Check sheet for the modelled part. Datum: model origin and axes. Units: mm. A direction names the side the tool comes from. Coordinates: 2 decimals unless noted, no trailing zeros. Order: outer loops, then holes, each group sorted by start corner. A loop starts at its lowest first (then second) coordinate and runs counter-clockwise, first axis right, second up.
from build123d import *

# Parameters (mm, degrees)
F0_W     = 115
F0_H     = 67
F1_DEPTH = 52
F2_T     = -2
F3_R     = 3
F5_DEPTH = 115
F6_W     = 25
F6_H     = 15
F7_DEPTH = 2
F9_DEPTH = 2


with BuildPart() as f1:
    # F0 (on Top) → F1 (new body)
    with BuildSketch(Plane.XY):
        Rectangle(F0_W, F0_H)
    extrude(amount=F1_DEPTH)

    # F2
    f2_openings = [f1.faces().sort_by_distance(p)[0] for p in [
        (0, 0, 52),
    ]]
    offset(amount=F2_T, openings=f2_openings)

    # F3
    f3_edges = [f1.edges().sort_by_distance(p)[0] for p in [
        (57.5, 33.5, 26),
        (57.5, -33.5, 26),
        (-57.5, -33.5, 26),
        (-57.5, 33.5, 26),
        (-57.5, 0, 0),
        (0, -33.5, 0),
        (0, 33.5, 0),
        (57.5, 0, 0),
    ]]
    fillet(f3_edges, radius=F3_R)

    # F4 (on face) → F5 (cut, through all)
    with BuildSketch(Plane(origin=(-57.5, 0, 0), x_dir=(0, -1, 0), z_dir=(-1, 0, 0))):
        with BuildLine():
            Line((-8.5, 52), (-18.5, 52))
            Line((-18.5, 52), (-18.5, 37))
            ThreePointArc((-18.5, 37), (-8.5, 27), (1.5, 37))
            Line((1.5, 37), (1.5, 52))
            Line((1.5, 52), (-8.5, 52))
        make_face()
    extrude(amount=-F5_DEPTH, mode=Mode.SUBTRACT)

    # F6 (on face) → F7 (cut, through all)
    with BuildSketch(Plane.YZ.offset(57.5)):
        with Locations((-14, 44.5)):
            Rectangle(F6_W, F6_H)
    extrude(amount=-F7_DEPTH, mode=Mode.SUBTRACT)

    # F8 (on face) → F9 (cut, through all)
    with BuildSketch(Plane.XZ.offset(33.5)):
        with BuildLine():
            Line((46, 52), (33, 52))
            Line((33, 52), (33, 43))
            ThreePointArc((33, 43), (33.5857864376, 41.5857864376), (35, 41))
            Line((35, 41), (44, 41))
            ThreePointArc((44, 41), (45.4142135624, 41.5857864376), (46, 43))
            Line((46, 43), (46, 52))
        make_face()
    extrude(amount=-F9_DEPTH, mode=Mode.SUBTRACT)


solid = f1.part
(1) Release check for a two-part mould opening along Y. For faces 3 (the flat face through (-55.5, 0, 27)), 4 (the cylindrical face through (56.6, -32.64, 27.84)), 5 (the flat face through (53, -32, 52)) record: +Y half, -Y half, draft (parallel to the pull), parting line (faces both ways), or undercut.
Filled in:
face 3: undercut
face 4: -Y half
face 5: draft
(2) Tool access check on faces 1 (the flat face through (-1, 0, 2)), 2 (the cylindrical face through (56.5, 8.7, 27)). Record the directions out of +Z, -Z, +X, -X, +Y, -Y that give a thin tool (end or side, any length) a straight path to the whole face; none if there is none.
Filled in:
face 1: +Z
face 2: +Z, +X, -X
(3) Thickness scan on probe 1 along X at (y, z) = (17.5, 18); probe 2 along Y at (x, z) = (-35.5, 37); probe 3 along X at (y, z) = (-15, 40.5). Record the ranges inside material, lowest first.
Filled in:
probe 1: x = -57.5 to -55.5, 55.5 to 57.5
probe 2: y = -33.5 to -31.5, 31.5 to 33.5
probe 3: x = -57.5 to -55.5
(4) Go/stop test with flat-tipped pins: P1, Ø15, axis at y = 10.5, z = 37, coming from the +X side; P2, Ø1.6, axis at y = -32.5, z = 46, coming from the -X side; P3, Ø0.6, axis at x = -56, z = 41, coming from the +Y side; P4, Ø2, axis at y = -32, z = 47.5, coming from the +X side. Record where each tip stops, or that it passes through.
Filled in:
P1: passes through
P2: stops at x = -57.25
P3: stops at y = 33.25
P4: stops at x = 57.46
(5) Cross-section at B-B (x = 41). Enter the section's corners in (y, z).
Filled in:
outline: (-33.5, 3) arc R3 ccw to (-30.5, 0) - (30.5, 0) arc R3 ccw to (33.5, 3) - (33.5, 52) - (31.5, 52) - (31.5, 2) - (-31.5, 2) - (-31.5, 41) - (-33.5, 41) - close
(6) Cross-section at A-A (z = 25). Enter the section's corners in (x, y).
Filled in:
outline: (-57.5, -30.5) arc R3 ccw to (-54.5, -33.5) - (54.5, -33.5) arc R3 ccw to (57.5, -30.5) - (57.5, 30.5) arc R3 ccw to (54.5, 33.5) - (-54.5, 33.5) arc R3 ccw to (-57.5, 30.5) - close; hole (-55.5, -31.5) - (55.5, -31.5) - (55.5, 31.5) - (-55.5, 31.5) - close
(7) Cross-section at D-D (z = 34). Enter the section's corners in (x, y), and give its area (3 significant figures).
Filled in:
outline: (-57.5, -30.5) arc R3 ccw to (-54.5, -33.5) - (54.5, -33.5) arc R3 ccw to (57.5, -30.5) - (57.5, -1.04) - (55.5, -1.04) - (55.5, -31.5) - (-55.5, -31.5) - (-55.5, -1.04) - (-57.5, -1.04) - close; (-57.5, 18.04) - (-55.5, 18.04) - (-55.5, 31.5) - (55.5, 31.5) - (55.5, 18.04) - (57.5, 18.04) - (57.5, 30.5) arc R3 ccw to (54.5, 33.5) - (-54.5, 33.5) arc R3 ccw to (-57.5, 30.5) - close
area: 628 mm2
(8) Cross-section at C-C (y = 8.5). Enter the section's corners in (x, z).
Filled in:
outline: (-57.5, 3) arc R3 ccw to (-54.5, 0) - (54.5, 0) arc R3 ccw to (57.5, 3) - (57.5, 27) - (55.5, 27) - (55.5, 2) - (-55.5, 2) - (-55.5, 27) - (-57.5, 27) - close
